```python
from build123d import *

# Parameters (mm, degrees)
F1_DEPTH = 30.7
F2_R     = 2
F3_DEPTH = 6
F2_W     = 34
F2_H     = 11
F4_DEPTH = 4
F5_SIZE  = 0.5


with BuildPart() as f1:
    # F0 (on Front) → F1 (new body, symmetric)
    with BuildSketch(Plane.XZ):
        Polygon((-17, 0), (-7.5, 0), (-5.3786796564, 2.1213203436), (-5.3786796564, 5.1213203436), (-7.5, 7.2426406871), (-7.5, 8.2426406871), (-5.0426406871, 10.7), (5.0426406871, 10.7), (7.5, 8.2426406871), (7.5, 7.2426406871), (5.3786796564, 5.1213203436), (5.3786796564, 2.1213203436), (7.5, 0), (17, 0), (17, 23.7), (-17, 23.7), align=None)
    extrude(amount=F1_DEPTH, both=True)

    # F2 (on face) → F3 (cut)
    with BuildSketch(Plane.XY.offset(23.7)):
        with Locations((-13, 13)):
            Circle(F2_R)
        with Locations((13, 13)):
            Circle(F2_R)
        with Locations((13, -13)):
            Circle(F2_R)
        with Locations((-13, -13)):
            Circle(F2_R)
    extrude(amount=-F3_DEPTH, mode=Mode.SUBTRACT)

    # F2 (on face) → F4 (cut)
    with BuildSketch(Plane.XY.offset(23.7)):
        with Locations((0, 25.2)):
            Rectangle(F2_W, F2_H)
        with Locations((0, -25.2)):
            Rectangle(F2_W, F2_H)
    extrude(amount=-F4_DEPTH, mode=Mode.SUBTRACT)

    # F5
    f5_edges = [f1.edges().sort_by_distance(p)[0] for p in [
        (17, 0, 0),
        (-17, 0, 0),
        (0, -30.7, 19.7),
        (-17, -25.2, 19.7),
        (17, -30.7, 9.85),
        (-17, -30.7, 9.85),
        (0, 30.7, 19.7),
        (17, 30.7, 9.85),
        (-17, 30.7, 9.85),
        (12.25, 30.7, 0),
        (-12.25, 30.7, 0),
        (-12.25, -30.7, 0),
        (12.25, -30.7, 0),
        (17, -25.2, 19.7),
        (-17, 25.2, 19.7),
        (17, 25.2, 19.7),
    ]]
    chamfer(f5_edges, length=F5_SIZE)


solid = f1.part
```
Read the model definition and answer for the solid it produces. Units are mm, in the model's axes. A direction names the side the tool comes from. Coordinates: 2 decimals unless noted, no trailing zeros. Order: outer loops, then holes, each group sorted by start corner. A loop starts at its lowest first (then second) coordinate and runs counter-clockwise, first axis right, second up. Notation, with made-up numbers: (-37, -1) - (-27, -1) arc R25 cw to (-27, 31) - close; hole circle Ø1 at (-15.5, -21.5). An arc over 180 degrees is marked (long way). Answer as a JSON object with one key per item and string values. Group by question number.
Item 1: Section D-D (x = -10) is taken. Give the vertices of the cut face in (y, z), plus the area to 3 significant figures.
Item 2: Consider probe 1 along Y at (x, z) = (-13, 19.1); probe 2 along Y at (x, z) = (13, 21.85); probe 3 along X at (y, z) = (21, 4.5). Determine where each line is inside the solid, lowest interval first. Write a range as from..to.
Item 3: A tool of negligible diameter and unlimited length cuts with its end or side. For faces 5 (the face through (5.379, 0, 4)), 6 (the face through (6.454, -0.43, 6.197)), 7 (the face through (13, 13, 17.7)), from which of +Z, -Z, +X, -X, +Y, -Y can it reach the whole face along a straight path? Write none if from no direction.
Item 4: Section B-B (y = -17.5) is taken. Give the vertices of the cut face in (x, z).
Item 5: Flat-ended cylindrical pins translate along their axes: P1, Ø5, axis at x = 13, y = -13, coming from the +Z side; P2, Ø2, axis at x = 13, y = -12.5, coming from the +Z side; P3, Ø3, axis at x = -2, y = 5, coming from the -Z side; P4, Ø5, axis at x = -6, y = -23.5, coming from the +Z side. Find the tip coordinate at first contact, or state that the pin passes through.
Item 6: Section C-C (z = 21) is taken. Give the vertices of the cut face in (x, y), plus the area to 3 significant figures.
Item 7: Section A-A (z = 3) is taken. Give the vertices of the cut face in (x, y).
Item 8: The mould has two halves that part along Z. Classify faces 1 (the face through (-13, -13, 17.7)), 2 (the face through (0, 19.7, 22)), 3 (the face through (-6.29, -0.43, 9.45)), 4 (the face through (-6.424, -0.43, 6.167)): +Z half, -Z half, draft (parallel to the pull), parting line (faces both ways), or undercut.
Results are:
{
 "1": {"outline": "(-30.7, 0.5) - (-30.2, 0) - (30.2, 0) - (30.7, 0.5) - (30.7, 19.2) - (30.2, 19.7) - (19.7, 19.7) - (19.7, 23.7) - (-19.7, 23.7) - (-19.7, 19.7) - (-30.2, 19.7) - (-30.7, 19.2) - close", "area": "1,370 mm^2"},
 "2": {"probe 1": "y = -30.7..-15, -11..11, 15..30.7", "probe 2": "y = -19.7..-15, -11..11, 15..19.7", "probe 3": "x = -17..-5.38, 5.38..17"},
 "3": {"face 5": "-Z, +Y, -Y", "face 6": "+Y, -Y", "face 7": "+Z"},
 "4": {"outline": "(-17, 0.5) - (-16.5, 0) - (-7.5, 0) - (-5.38, 2.12) - (-5.38, 5.12) - (-7.5, 7.24) - (-7.5, 8.24) - (-5.04, 10.7) - (5.04, 10.7) - (7.5, 8.24) - (7.5, 7.24) - (5.38, 5.12) - (5.38, 2.12) - (7.5, 0) - (16.5, 0) - (17, 0.5) - (17, 23.7) - (-17, 23.7) - close"},
 "5": {"P1": "stops at z = 23.7", "P2": "stops at z = 17.7", "P3": "stops at z = 10.7", "P4": "stops at z = 19.7"},
 "6": {"outline": "(-17, -19.7) - (17, -19.7) - (17, 19.7) - (-17, 19.7) - close; hole circle Ø4 at (-13, -13); hole circle Ø4 at (-13, 13); hole circle Ø4 at (13, -13); hole circle Ø4 at (13, 13)", "area": "1,290 mm^2"},
 "7": {"outline": "(-17, -30.2) - (-16.5, -30.7) - (-5.38, -30.7) - (-5.38, 30.7) - (-16.5, 30.7) - (-17, 30.2) - close; (5.38, -30.7) - (16.5, -30.7) - (17, -30.2) - (17, 30.2) - (16.5, 30.7) - (5.38, 30.7) - close"},
 "8": {"face 1": "+Z half", "face 2": "draft", "face 3": "undercut", "face 4": "undercut"}
}
